Could you check a few things on this drawing? It's one solid part, dimensions in mm from its lowest x, y, z. A direction names the side the tool comes from. Give positions to 0.01 mm unless a question says otherwise; leave off trailing zeros. Write each loop counter-clockwise with the first axis right and the second up, starting at its lowest first coordinate (ties: lowest second). Pieces come first, ordered by that corner, then holes. Notation, with made-up numbers: (-20.75, 26.5) -> (19.25, 26.5) arc R9 ccw to (19.25, 34.5) -> close; hole circle Ø4 at (-16.75, 57). An arc over 180 degrees is marked (long way). Answer as CSV lines item,"result". Start each with the question number.
1. On a 3-axis mill with a long thin cutter (end or side, diameter ignored), from which of +Z, -Z, +X, -X, +Y, -Y can I reach the whole of each face in a straight line? I mean the marked faces 1 and 2. Say none if no direction works.
2. If we section it at B-B on z = 6.5: Write out the boundary of the cut face in (x, y) (3 decimals).
3. I'm going to push flat-ended pins straight in: P1, Ø5, axis at x = 193.5, z = 6.5, coming from the -Y side; P2, Ø5, axis at y = 103, z = 5.5, coming from the -X side. Where does each tip first touch, or does it pass through?
4. I need wall thicknesses on line 1 (Y direction, x = 25.4, z = 19) (3 decimals); line 2 (Y direction, x = 234.95, z = 19.75) (3 decimals); line 3 (Y direction, x = 108, z = 11.25). Which ranges of each line are inside material? Lowest first, please. Write a range as [from, to].
5. If we section it at D-D on x = 136: Write out the boundary of the cut face in (y, z).
6. If we section it at A-A on y = 133.35: Write out the boundary of the cut face in (x, z) (3 decimals).
7. If we section it at C-C on x = 234.95: Write out the boundary of the cut face in (y, z) (3 decimals).
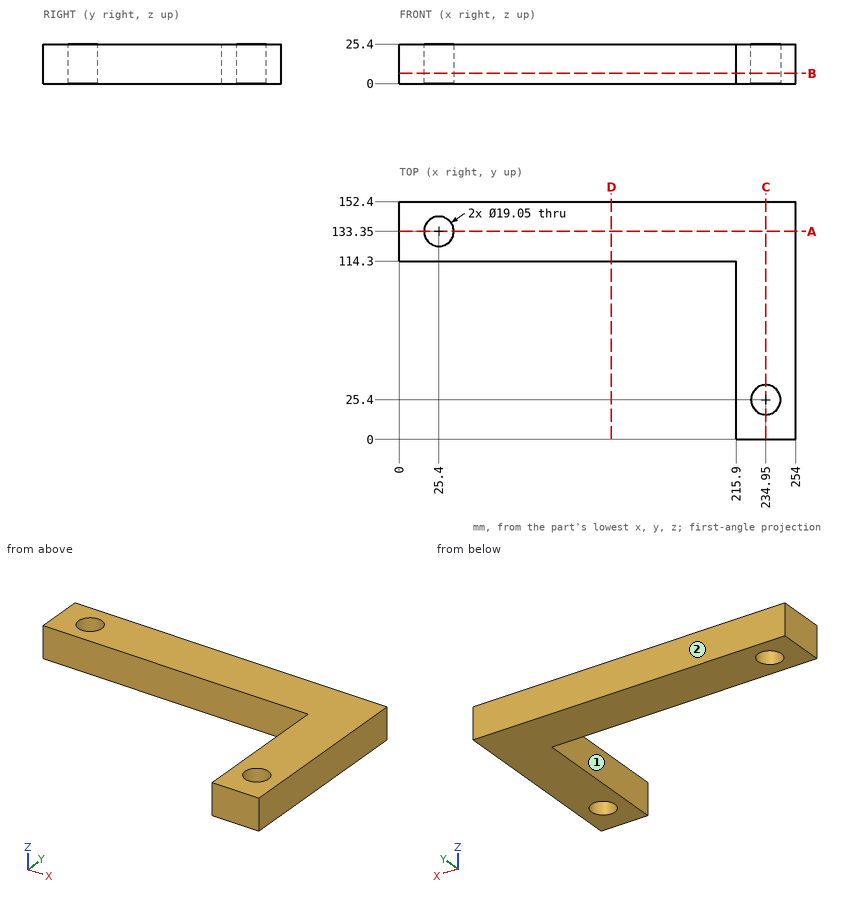
Computed values:
1,face 1,"+Z, -Z, -X, -Y"
1,face 2,"+Z, -Z, +X, -X, +Y"
2,outline,"(0, 114.3) -> (215.9, 114.3) -> (215.9, 0) -> (254, 0) -> (254, 152.4) -> (0, 152.4) -> close; hole circle Ø19.05 at (25.4, 133.35); hole circle Ø19.05 at (234.95, 25.4)"
3,P1,"stops at y = 114.3"
3,P2,"stops at x = 215.9"
4,line 1,"y = [114.3, 123.825], [142.875, 152.4]"
4,line 2,"y = [0, 15.875], [34.925, 152.4]"
4,line 3,"y = [114.3, 152.4]"
5,outline,"(114.3, 0) -> (152.4, 0) -> (152.4, 25.4) -> (114.3, 25.4) -> close"
6,outline,"(0, 0) -> (15.875, 0) -> (15.875, 25.4) -> (0, 25.4) -> close; (34.925, 0) -> (254, 0) -> (254, 25.4) -> (34.925, 25.4) -> close"
7,outline,"(0, 0) -> (15.875, 0) -> (15.875, 25.4) -> (0, 25.4) -> close; (34.925, 0) -> (152.4, 0) -> (152.4, 25.4) -> (34.925, 25.4) -> close"
